Read the model definition and answer for the solid it produces. Units are mm, in the model's axes. Coordinates: 2 decimals unless noted, no trailing zeros. Write each loop counter-clockwise with the first axis right and the second up, starting at its lowest first coordinate (ties: lowest second). Pieces come first, ordered by that corner, then holes. Notation, with made-up numbers: (25, 76) - (31, 76) arc R32 cw to (31, 109) - close; hole circle Ø6 at (56.5, -15). An arc over 180 degrees is marked (long way). Use a Markdown table: item, result.
from build123d import *

# Parameters (mm, degrees)
SKETCH_1_W          = 160
SKETCH_1_H          = 130
EXTRUDE_1_DEPTH     = 4
SKETCH_2_R          = 1.75
CUT_EXTRUDE_1_DEPTH = 5
SKETCH_4_R          = 1.75
CUT_EXTRUDE_2_DEPTH = 5
SKETCH_5_R          = 1.75
CUT_EXTRUDE_3_DEPTH = 5
SKETCH_6_R          = 1.75
CUT_EXTRUDE_4_DEPTH = 5
SKETCH_7_W          = 33
SKETCH_7_H          = 39
EXTRUDE_2_DEPTH     = 4
SKETCH_8_R          = 1.75
CUT_EXTRUDE_5_DEPTH = 5
FILLET_1_R          = 10
FILLET_2_R          = 5
SKETCH_9_R          = 1.75
CUT_EXTRUDE_6_DEPTH = 5


with BuildPart() as part:
    # ｽｹｯﾁ1 → ﾎﾞｽ - 押し出し1 (new body)
    with BuildSketch(Plane(origin=(0, 0, 0), x_dir=(1, 0, 0), z_dir=(0, 1, 0))):
        Rectangle(SKETCH_1_W, SKETCH_1_H)
    extrude(amount=EXTRUDE_1_DEPTH)

    # ｽｹｯﾁ2 → ｶｯﾄ - 押し出し1 (cut, through all)
    with BuildSketch(Plane(origin=(0, 4, 0), x_dir=(1, 0, 0), z_dir=(0, 1, 0))):
        with Locations((-73, -15)):
            Circle(SKETCH_2_R)
        with Locations((-73, 51)):
            Circle(SKETCH_2_R)
        with Locations((-46, -15)):
            Circle(SKETCH_2_R)
        with Locations((-46, 51)):
            Circle(SKETCH_2_R)
    extrude(amount=-CUT_EXTRUDE_1_DEPTH, mode=Mode.SUBTRACT)

    # ｽｹｯﾁ4 → ｶｯﾄ - 押し出し2 (cut, through all)
    with BuildSketch(Plane(origin=(0, 4, 0), x_dir=(1, 0, 0), z_dir=(0, 1, 0))):
        with Locations((41, 59)):
            Circle(SKETCH_4_R)
        with Locations((41, 32)):
            Circle(SKETCH_4_R)
    extrude(amount=-CUT_EXTRUDE_2_DEPTH, mode=Mode.SUBTRACT)

    # ｽｹｯﾁ5 → ｶｯﾄ - 押し出し3 (cut, through all)
    with BuildSketch(Plane(origin=(0, 4, 0), x_dir=(1, 0, 0), z_dir=(0, 1, 0))):
        with Locations((57, -61)):
            Circle(SKETCH_5_R)
        with Locations((-20, -61)):
            Circle(SKETCH_5_R)
        with Locations((-39, -32)):
            Circle(SKETCH_5_R)
        with Locations((76, -32)):
            Circle(SKETCH_5_R)
        with Locations((28.5, 29)):
            Circle(SKETCH_5_R)
    extrude(amount=-CUT_EXTRUDE_3_DEPTH, mode=Mode.SUBTRACT)

    # ｽｹｯﾁ6 → ｶｯﾄ - 押し出し4 (cut, through all)
    with BuildSketch(Plane(origin=(0, 4, 0), x_dir=(1, 0, 0), z_dir=(0, 1, 0))):
        with Locations((0, 55)):
            Circle(SKETCH_6_R)
        with Locations((0, 40)):
            Circle(SKETCH_6_R)
        with Locations((15, 55)):
            Circle(SKETCH_6_R)
        with Locations((15, 40)):
            Circle(SKETCH_6_R)
        with Locations((-15, 55)):
            Circle(SKETCH_6_R)
        with Locations((-15, 40)):
            Circle(SKETCH_6_R)
    extrude(amount=-CUT_EXTRUDE_4_DEPTH, mode=Mode.SUBTRACT)

    # ｽｹｯﾁ7 → ﾎﾞｽ - 押し出し2 (add)
    with BuildSketch(Plane(origin=(0, 4, 0), x_dir=(1, 0, 0), z_dir=(0, 1, 0))):
        with Locations((96.5, 45.5)):
            Rectangle(SKETCH_7_W, SKETCH_7_H)
    extrude(amount=-EXTRUDE_2_DEPTH)

    # ｽｹｯﾁ8 → ｶｯﾄ - 押し出し5 (cut, through all)
    with BuildSketch(Plane(origin=(0, 4, 0), x_dir=(1, 0, 0), z_dir=(0, 1, 0))):
        with Locations((107, 59)):
            Circle(SKETCH_8_R)
        with Locations((107, 32)):
            Circle(SKETCH_8_R)
    extrude(amount=-CUT_EXTRUDE_5_DEPTH, mode=Mode.SUBTRACT)

    # ﾌｨﾚｯﾄ1
    fillet_1_edges = [part.edges().sort_by_distance(p)[0] for p in [
        (80, 2, 65),
        (-80, 2, 65),
        (-80, 2, -65),
        (80, 2, -26),
    ]]
    fillet(fillet_1_edges, radius=FILLET_1_R)

    # ﾌｨﾚｯﾄ2
    fillet_2_edges = [part.edges().sort_by_distance(p)[0] for p in [
        (113, 2, -65),
        (113, 2, -26),
    ]]
    fillet(fillet_2_edges, radius=FILLET_2_R)

    # ｽｹｯﾁ9 → ｶｯﾄ - 押し出し6 (cut, through all)
    with BuildSketch(Plane(origin=(0, 4, 0), x_dir=(1, 0, 0), z_dir=(0, 1, 0))):
        with Locations((-65, -50)):
            Circle(SKETCH_9_R)
        with Locations((-50, -50)):
            Circle(SKETCH_9_R)
        with Locations((-65, -35)):
            Circle(SKETCH_9_R)
        with Locations((-50, -35)):
            Circle(SKETCH_9_R)
    extrude(amount=-CUT_EXTRUDE_6_DEPTH, mode=Mode.SUBTRACT)


solid = part.part
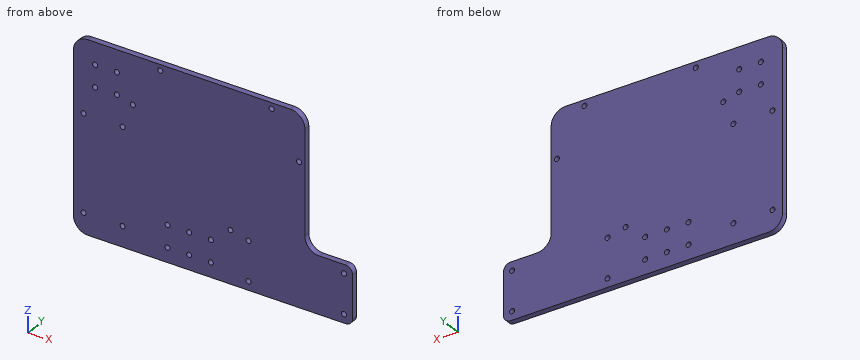
(1) Each of these flat-tipped pins is pushed along its axis until it touches: P1, Ø4.5, axis at x = 41, z = -59, coming from the -Y side; P2, Ø2, axis at x = 28.5, z = -29, coming from the +Y side. Where does it stop, or does it pass through?
Report:
| item | result |
|---|---|
| P1 | stops at y = 0 |
| P2 | passes through |
(2) A cutting plane is placed at A-A, the plane x = 84. Write down the section's boundary in (y, z).
Report:
| item | result |
|---|---|
| outline | (0, -65) - (4, -65) - (4, -24) - (0, -24) - close |
(3) A cutting plane is placed at B-B, the plane z = 9.5. Write down the section's boundary in (x, y).
Report:
| item | result |
|---|---|
| outline | (-80, 0) - (80, 0) - (80, 4) - (-80, 4) - close |
(4) Straight lines are drawn through the part: L1, parallel to Z at x = -50, y = 2.85; L2, parallel to X at y = 2.15, z = -40; L3, parallel to X at y = 2.85, z = 50. For each, find the intervals that lie inside material, in ascending order.
Report:
| item | result |
|---|---|
| L1 | z = -65 to 33.25, 36.75 to 48.25, 51.75 to 65 |
| L2 | x = -80 to -16.75, -13.25 to -1.75, 1.75 to 13.25, 16.75 to 113 |
| L3 | x = -80 to -66.75, -63.25 to -51.75, -48.25 to 80 |
